```python
from build123d import *

# Parameters (mm, degrees)
PAD102_DEPTH      = 16
SKETCH199_R       = 1.75
POCKET_DEPTH      = 9.701
POCKET_DEPTH_BACK = 5.001
SKETCH200_R       = 3.25
POCKET073_DEPTH   = 10.001


with BuildPart() as part:
    # Sketch198 → Pad102 (new body, symmetric)
    with BuildSketch(Plane.XZ):
        with BuildLine():
            ThreePointArc((-7.5, -30.5), (-7.146447, -30.353554), (-7, -30))
            Line((-7, -30), (-7, -25.010349))
            ThreePointArc((-7, -25.010349), (-6.640965, -24.242779), (-5.821673, -24.026377))
            Line((-5.821673, -24.026377), (-0.891634, -24.919857))
            ThreePointArc((-0.891634, -24.919857), (5, -19.998107), (-0.89536, -15.08082))
            Line((-0.89536, -15.08082), (-5.820928, -15.977343))
            ThreePointArc((-5.820928, -15.977343), (-6.640675, -15.76132), (-7, -14.993507))
            Line((-7, -14.993507), (-7, -11))
            ThreePointArc((-7, -11), (-7.146447, -10.646447), (-7.5, -10.5))
            Line((-7.5, -10.5), (-9.7, -10.5))
            Line((-9.7, -10.5), (-9.7, -30.5))
            Line((-9.7, -30.5), (-7.5, -30.5))
        make_face()
    extrude(amount=PAD102_DEPTH, both=True)

    # Sketch199 → Pocket (cut, two sides)
    with BuildSketch(Plane.YZ) as pocket_sk:
        with Locations((0, -20)):
            Circle(SKETCH199_R)
    extrude(amount=-POCKET_DEPTH, mode=Mode.SUBTRACT)
    extrude(pocket_sk.sketch, amount=POCKET_DEPTH_BACK, mode=Mode.SUBTRACT)

    # Sketch200 → Pocket073 (cut, through all)
    with BuildSketch(Plane.YZ.offset(-5)):
        with Locations((0, -20)):
            Circle(SKETCH200_R)
    extrude(amount=POCKET073_DEPTH, mode=Mode.SUBTRACT)


solid = part.part
```
CAD build for the part. Positions are in the model's coordinates, mm. A direction names the side the tool comes from. Give positions to 0.01 mm unless a question says otherwise; leave off trailing zeros. Loops run counter-clockwise (first coordinate to the right, second up) from the corner with the lowest first, then second, coordinate; pieces in that order, holes last. Notation, with made-up numbers: (-33, 82.25) -> (-26, 82.25) arc R23 ccw to (-26, 117.25) -> close; hole circle Ø6 at (2, 33.5). An arc over 180 degrees is marked (long way). Use a Markdown table: item, result.
1. Wall check: L1, parallel to Y at x = 1.25, z = -20; L2, parallel to Z at x = -7.6, y = 0; L3, parallel to Z at x = -6, y = 0. Give the ranges that are in metal, low to high. Write a range as [from, to].
Check result:
| item | result |
|---|---|
| L1 | y = [-16, -3.25], [3.25, 16] |
| L2 | z = [-30.5, -21.75], [-18.25, -10.5] |
| L3 | z = [-24.01, -21.75], [-18.25, -15.99] |
2. Which spindle directions (+Z, -Z, +X, -X, +Y, -Y) get a long thin tool onto all of the face, cutting with end or side? Do faces 1 (the flat face through (-3.324, -0.224, -15.523)), 2 (the flat face through (-7, 0, -13)), 3 (the cylindrical face through (-0.066, -3.247, -19.857)). Say none if no direction does.
Check result:
| item | result |
|---|---|
| face 1 | +Z, +Y, -Y |
| face 2 | +Z, +X, +Y, -Y |
| face 3 | +X |
3. Slice it at B-B (y = 0). List the corners of the cut face in (x, z), plus the area to 3 significant figures.
Check result:
| item | result |
|---|---|
| outline | (-9.7, -30.5) -> (-7.5, -30.5) arc R0.5 ccw to (-7, -30) -> (-7, -25.01) arc R1 cw to (-5.82, -24.03) -> (-0.89, -24.92) arc R5 ccw to (3.8, -23.25) -> (-5, -23.25) -> (-5, -21.75) -> (-9.7, -21.75) -> close; (-9.7, -18.25) -> (-5, -18.25) -> (-5, -16.75) -> (3.8, -16.75) arc R5 ccw to (-0.9, -15.08) -> (-5.82, -15.98) arc R1 cw to (-7, -14.99) -> (-7, -11) arc R0.5 ccw to (-7.5, -10.5) -> (-9.7, -10.5) -> close |
| area | 77.0 mm^2 |
4. Flat gauge pins, fed straight in: pin 1 (1 mm diameter, centred on y = 0, z = -17.5, fed in from +X); pin 2 (3 mm diameter, centred on y = 4, z = -12.5, fed in from +X); pin 3 (2 mm diameter, centred on y = 0, z = -20, fed in from +X); pin 4 (1 mm diameter, centred on x = -5, y = 2.5, fed in from +Z). Where does each tip first touch, or does it go through?
Check result:
| item | result |
|---|---|
| pin 1 | stops at x = -5 |
| pin 2 | stops at x = -7 |
| pin 3 | passes through |
| pin 4 | stops at z = -15.74 |
5. Slice it at C-C (x = 4.25). List the corners of the cut face in (y, z).
Check result:
| item | result |
|---|---|
| outline | (-16, -22.63) -> (-1.9, -22.63) arc R3.25 cw to (-1.9, -17.37) -> (-16, -17.37) -> close; (1.9, -22.63) -> (16, -22.63) -> (16, -17.37) -> (1.9, -17.37) arc R3.25 cw to start |
6. Slice it at A-A (z = -20). List the corners of the cut face in (x, y).
Check result:
| item | result |
|---|---|
| outline | (-9.7, -16) -> (5, -16) -> (5, -3.25) -> (-5, -3.25) -> (-5, -1.75) -> (-9.7, -1.75) -> close; (-9.7, 1.75) -> (-5, 1.75) -> (-5, 3.25) -> (5, 3.25) -> (5, 16) -> (-9.7, 16) -> close |
7. Mould opens along X. For faces 4 (the cylindrical face through (-6.63, -0.22, -15.77)), 5 (the flat face through (-7, 0, -28)), 6 (the flat face through (-9, 0, -30.5)), 7 (the flat face through (-3.391, -0.224, -24.467)) say: pulls with the +X half, pulls with the -X half, needs draft (parallel to the pull), parting line crosses it, or undercut.
Check result:
| item | result |
|---|---|
| face 4 | undercut |
| face 5 | pulls with the +X half |
| face 6 | needs draft |
| face 7 | undercut |
8. Slice it at D-D (y = -9.5). List the corners of the cut face in (x, z).
Check result:
| item | result |
|---|---|
| outline | (-9.7, -30.5) -> (-7.5, -30.5) arc R0.5 ccw to (-7, -30) -> (-7, -25.01) arc R1 cw to (-5.82, -24.03) -> (-0.89, -24.92) arc R5 ccw (long way) to (-0.9, -15.08) -> (-5.82, -15.98) arc R1 cw to (-7, -14.99) -> (-7, -11) arc R0.5 ccw to (-7.5, -10.5) -> (-9.7, -10.5) -> close |
